```python
from build123d import *

# Parameters (mm, degrees)
F1_DEPTH      = 19.05
F4_DEPTH      = 11.43
F8_W          = 58.2950823009
F8_H          = 18.0758163333
F9_DEPTH      = 19.051
F9_DEPTH_BACK = 11.74174
F11_W         = 68.613074236
F11_H         = 25.4
F12_DEPTH     = 2.54
F13_W         = 19.8203250766
F13_H         = 44.8987269774
F14_DEPTH     = 7.62


with BuildPart() as f1:
    # F0 (on Front) → F1 (new body, symmetric)
    with BuildSketch(Plane.XZ):
        with BuildLine():
            Line((16.493462882, 12.7), (-77.7931159433, 2.3487282923))
            ThreePointArc((-77.7931159433, 2.3487282923), (-79.6990393329, 1.6031312535), (-80.9712142796, 0))
            Line((-80.9712142796, 0), (50.8, 0))
            Line((50.8, 0), (50.8, 12.7))
            Line((50.8, 12.7), (16.493462882, 12.7))
        make_face()
    extrude(amount=F1_DEPTH, both=True)

    # F3 (on offset) → F4 (cut)
    with BuildSketch(Plane.XY.offset(12.7)):
        with BuildLine():
            Line((-64.5951760395, -8.7044802925), (1.4448239605, -8.7044802925))
            ThreePointArc((1.4448239605, -8.7044802925), (10.3064292543, 0.1571250013), (1.4448239605, 9.0187302952))
            Line((1.4448239605, 9.0187302952), (-64.5951760395, 9.0187302952))
            ThreePointArc((-64.5951760395, 9.0187302952), (-73.4567813333, 0.1571250013), (-64.5951760395, -8.7044802925))
        make_face()
    extrude(amount=-F4_DEPTH, mode=Mode.SUBTRACT)

    # F5: F1 across plane


with BuildPart() as f1_1:
    add(f1.part)
    add(f1.part.mirror(Plane.XY))

    # F7: F1 across plane


with BuildPart() as f1_2:
    add(f1_1.part)
    add(f1_1.part.mirror(Plane.YZ.offset(50.8)))

    # F8 (on Front) → F9 (cut, two sides)
    with BuildSketch(Plane.XZ) as f9_sk:
        with Locations((50.8, 0)):
            Rectangle(F8_W, F8_H)
    extrude(amount=-F9_DEPTH, mode=Mode.SUBTRACT)
    extrude(f9_sk.sketch, amount=F9_DEPTH_BACK, mode=Mode.SUBTRACT)

    # F11 (on offset) → F12 (cut)
    with BuildSketch(Plane.XZ.offset(-19.05)):
        with Locations((50.8, 0)):
            Rectangle(F11_W, F11_H)
    extrude(amount=F12_DEPTH, mode=Mode.SUBTRACT)

    # F13 (on offset) → F14 (cut)
    with BuildSketch(Plane.XY.offset(12.7)):
        with Locations((67.3308186233, -3.4829550423)):
            Rectangle(F13_W, F13_H)
    extrude(amount=-F14_DEPTH, mode=Mode.SUBTRACT)


solid = f1_2.part
```
Geometry check sheet. Reference: the model listing, model coordinates, mm. A direction names the side the tool comes from. Give positions to 0.01 mm unless a question says otherwise; leave off trailing zeros. Loops run counter-clockwise (first coordinate to the right, second up) from the corner with the lowest first, then second, coordinate; pieces in that order, holes last. Notation, with made-up numbers: M 13.25,78.5 L 47.25,78.5 A29 cw 47.25,103.5 Z; hole C 27,31 d10. An arc over 180 degrees is marked long. Write item = value, one per line.
(1) Sectioned sample at A-A, the plane x = 30.5. Record the cut outline in (y, z).
Answer below:
outline = M -19.05,-12.7 L 16.51,-12.7 L 16.51,-9.04 L -11.74,-9.04 L -11.74,9.04 L 16.51,9.04 L 16.51,12.7 L -19.05,12.7 Z
(2) Material ranges on line 1 (Z direction, x = 38, y = 9); line 2 (Y direction, x = -39, z = 2.25); line 3 (Y direction, x = 65, z = -4.5), recorded low to high. Write a range as [from, to].
Answer below:
line_1 = [-12.7, -9.04], [9.04, 12.7]
line_2 = [-19.05, -8.7], [9.02, 19.05]
line_3 = [-19.05, -11.74]
(3) Sectioned sample at C-C, the plane y = -14. Record the cut outline in (x, z), plus the area to 3 significant figures.
Answer below:
outline = M -80.97,0 A3.93 ccw -77.79,-2.35 L 16.49,-12.7 L 85.11,-12.7 L 179.39,-2.35 A3.93 ccw 182.57,0 A3.93 ccw 179.39,2.35 L 85.11,12.7 L 77.24,12.7 L 77.24,5.08 L 57.42,5.08 L 57.42,12.7 L 16.49,12.7 L -77.79,2.35 A3.93 ccw Z
area = 4,450 mm2
(4) Release check for a two-part mould opening along Z. For faces 1 (the face through (125, 9.019, 5)), 2 (the face through (21.652, 2, 0)), 3 (the face through (50, -2, -12.7)) record: released by +Z, released by -Z, zero draft, split by the parting line, or undercut.
Answer below:
face_1 = zero draft
face_2 = undercut
face_3 = released by -Z
(5) Tool access check on faces 4 (the face through (50.6, 16.51, -9.3)), 5 (the face through (-73.455, 0.352, 2.271)), 6 (the face through (39, 2, 9.038)). Record the directions out of +Z, -Z, +X, -X, +Y, -Y that give a thin tool (end or side, any length) a straight path to the whole face; none if there is none.
Answer below:
face_4 = +Z, -Z, +Y
face_5 = +Z
face_6 = +Y
(6) Gauge pin test, flat ends, axial feed: pin 1 Ø10 at (x, y) = (98.5, -5) entering from -Z; pin 2 Ø2 at (x, y) = (-51, 9.5) entering from -Z; pin 3 Ø4 at (x, y) = (122.5, 0.5) entering from -Z. Record the tip position at first contact, or that the pin passes through.
Answer below:
pin_1 = -11.77
pin_2 = -5.4
pin_3 = -1.27
(7) Sectioned sample at B-B, the plane y = 13. Record the cut outline in (x, z), plus the area to 3 significant figures.
Answer below:
outline = M -80.97,0 A3.93 ccw -77.79,-2.35 L 16.49,-12.7 L 85.11,-12.7 L 179.39,-2.35 A3.93 ccw 182.57,0 A3.93 ccw 179.39,2.35 L 85.11,12.7 L 77.24,12.7 L 77.24,9.04 L 79.95,9.04 L 79.95,-9.04 L 21.65,-9.04 L 21.65,9.04 L 57.42,9.04 L 57.42,12.7 L 16.49,12.7 L -77.79,2.35 A3.93 ccw Z
area = 3,470 mm2
(8) Sectioned sample at D-D, the plane x = 117. Record the cut outline in (y, z).
Answer below:
outline = M -19.05,-9.2 L -8.7,-9.2 L -8.7,-1.27 L 9.02,-1.27 L 9.02,-9.2 L 19.05,-9.2 L 19.05,9.2 L 9.02,9.2 L 9.02,1.27 L -8.7,1.27 L -8.7,9.2 L -19.05,9.2 Z
